Answer from the drawing. Dimensions are ordinates in mm from the lowest x, y and z of the part. A direction names the side the tool comes from. Give positions to 0.01 mm unless a question says otherwise; leave off trailing zeros. Write each loop counter-clockwise with the first axis right and the second up, starting at its lowest first coordinate (ties: lowest second). Pieces come first, ordered by that corner, then holes. Notation, with made-up numbers: (36, 10) -> (81, 10) arc R10 cw to (81, 27) -> close; hole circle Ø11 at (-8.5, 50.5). An arc over 180 degrees is marked (long way). Use a Markdown table: item, result. Add a question column.
Q1. Consider line 1 (Z direction, x = 9.5, y = 3.3); line 2 (X direction, y = 3.4, z = 11); line 3 (Y direction, x = 7, z = 16.25). Determine where each line is inside the solid, lowest interval first.
Q2. For the marked faces 1 and 2, determine the directions among +Z, -Z, +X, -X, +Y, -Y from which every point of the face is accessible in a straight line to the end or side of a thin tool.
Q3. Section C-C, the plane y = 1.4 is taken. Give the vertices of the cut face in (x, z) (3 decimals).
Q4. Section B-B, the plane z = 3.5 is taken. Give the vertices of the cut face in (x, y) (3 decimals).
Q5. Section A-A, the plane x = 10.75 is taken. Give the vertices of the cut face in (y, z) (3 decimals).
Q6. Each of these flat-tipped pins is pushed along its axis until it touches: pin 1 Ø1.5 at (y, z) = (0.5, 3) entering from +X; pin 2 Ø7 at (x, z) = (9.525, 9.525) entering from +Y (3 decimals); pin 3 Ø1 at (y, z) = (1, 15) entering from -X. Where does it stop, or does it pass through?
Q7. Section D-D, the plane x = 6.75 is taken. Give the vertices of the cut face in (y, z) (3 decimals), plus the area to 3 significant figures.
Q8. For a pull along X with two mould halves and no side action, classify the marked faces 3, 4, 5 and 6 as pulls with the +X half, pulls with the -X half, needs draft (parallel to the pull), parting line crosses it, or undercut.
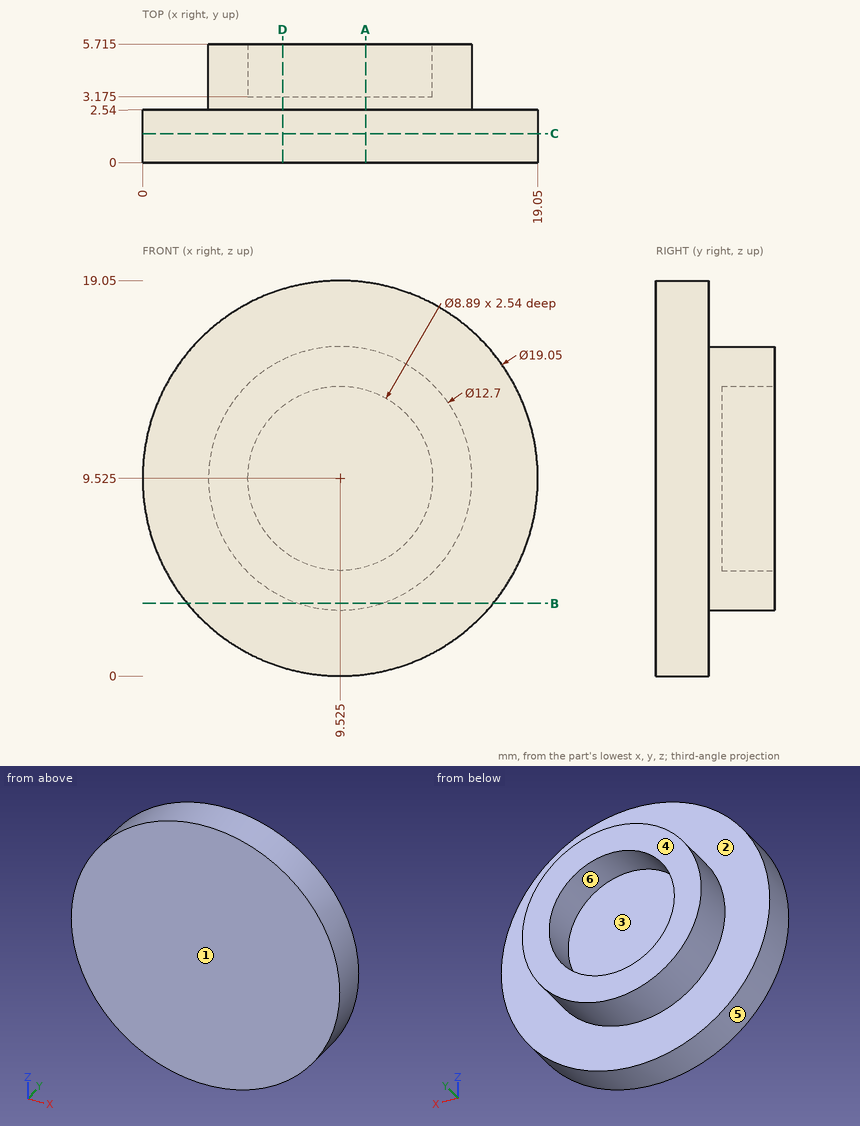
Result set:
| question | item | result |
|---|---|---|
| 1 | line 1 | z = 3.18 to 5.08, 13.97 to 15.87 |
| 1 | line 2 | x = 3.35 to 5.33, 13.72 to 15.7 |
| 1 | line 3 | y = 0 to 2.54 |
| 2 | face 1 | +Z, -Z, +X, -X, -Y |
| 2 | face 2 | +Y |
| 3 | outline | circle Ø19.05 at (9.525, 9.525) |
| 4 | outline | (2.148, 0) -> (16.902, 0) -> (16.902, 2.54) -> (11.53, 2.54) -> (11.53, 5.715) -> (7.52, 5.715) -> (7.52, 2.54) -> (2.148, 2.54) -> close |
| 5 | outline | (0, 0.079) -> (2.54, 0.079) -> (2.54, 3.294) -> (5.715, 3.294) -> (5.715, 5.252) -> (3.175, 5.252) -> (3.175, 13.798) -> (5.715, 13.798) -> (5.715, 15.756) -> (2.54, 15.756) -> (2.54, 18.971) -> (0, 18.971) -> close |
| 6 | pin 1 | stops at x = 17.1 |
| 6 | pin 2 | stops at y = 3.175 |
| 6 | pin 3 | stops at x = 1.4 |
| 7 | outline | (0, 0.413) -> (2.54, 0.413) -> (2.54, 3.813) -> (5.715, 3.813) -> (5.715, 6.053) -> (3.175, 6.053) -> (3.175, 12.997) -> (5.715, 12.997) -> (5.715, 15.237) -> (2.54, 15.237) -> (2.54, 18.637) -> (0, 18.637) -> close |
| 7 | area | 64.9 mm2 |
| 8 | face 3 | undercut |
| 8 | face 4 | needs draft |
| 8 | face 5 | parting line crosses it |
| 8 | face 6 | undercut |
